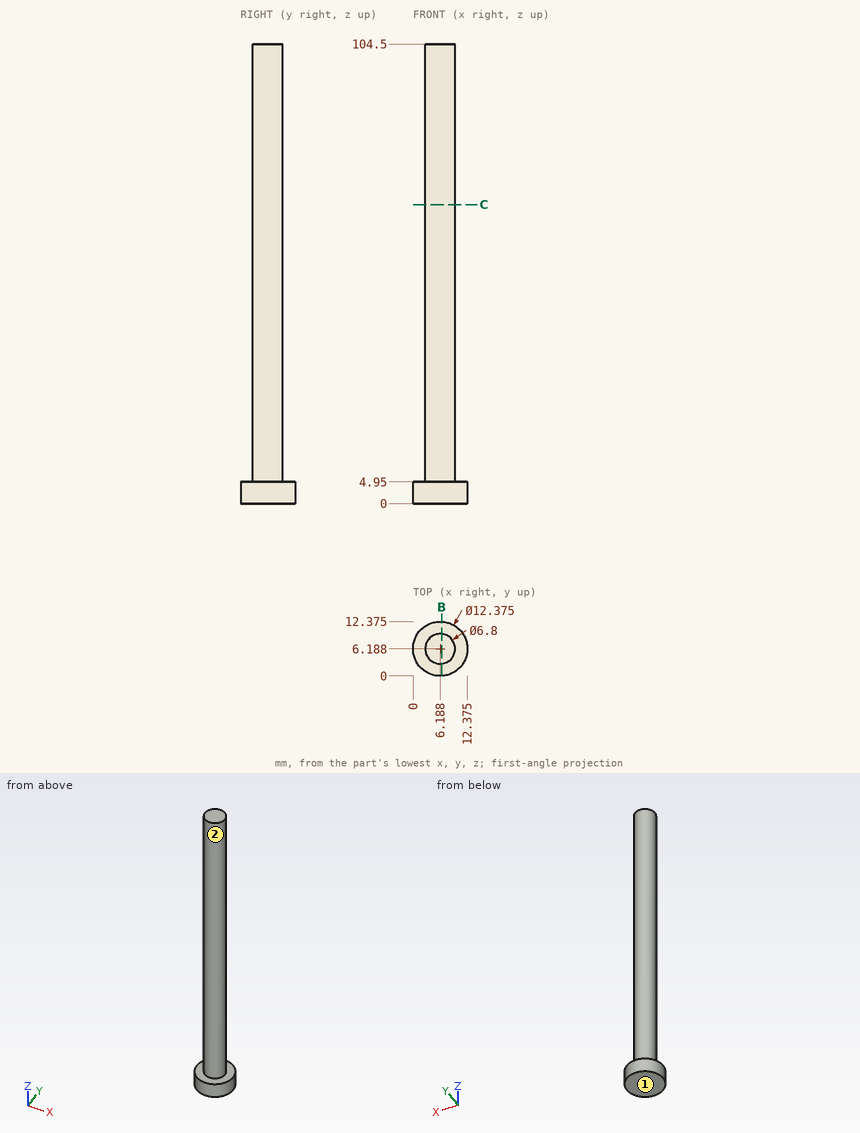
Geometry check sheet. Reference: drawing and pictorial views, mm from the part's lowest x, y, z. A direction names the side the tool comes from. Give positions to 0.01 mm unless a question says otherwise; leave off trailing zeros. Write each loop counter-clockwise with the first axis right and the second up, starting at its lowest first coordinate (ties: lowest second). Pieces come first, ordered by that corner, then holes. Notation, with made-up numbers: (-26, -12.5) -> (-3, -12.5) arc R25 cw to (-3, 0.5) -> close; hole circle Ø1 at (20, -33). An arc over 180 degrees is marked (long way). One line per item, written item: value. Start each with the question number.
Item 1: Section check C-C on z = 68. Record the cut outline in (x, y).
Item 2: Section check B-B on x = 6.5. Record the cut outline in (y, z), then the cut area to 3 significant figures.
Item 3: Material ranges on probe 1 along Z at (x, y) = (0.5, 7.25); probe 2 along X at (y, z) = (6.5, 62); probe 3 along X at (y, z) = (3.5, 66) (1 decimal), recorded low to high. Write a range as from..to.
Item 4: Gauge pin test, flat ends, axial feed: pin 1 (5 mm diameter, centred on x = 3.5, z = 33.5, fed in from +Y); pin 2 (3 mm diameter, centred on y = 6, z = 48, fed in from -X); pin 3 (6 mm diameter, centred on y = 1.5, z = 38.5, fed in from +X). Record the tip position at first contact, or that the pin passes through.
Item 5: Tool access check on the marked faces 1 and 2. Record the directions out of +Z, -Z, +X, -X, +Y, -Y that give a thin tool (end or side, any length) a straight path to the whole face; none if there is none.
Results list:
1. outline: circle Ø6.8 at (6.19, 6.19)
2. outline: (0.01, 0) -> (12.37, 0) -> (12.37, 4.95) -> (9.57, 4.95) -> (9.57, 104.5) -> (2.8, 104.5) -> (2.8, 4.95) -> (0.01, 4.95) -> close
2. area: 735 mm²
3. probe 1: 0..4.95
3. probe 2: 2.8..9.57
3. probe 3: 4.1..8.3
4. pin 1: y = 9.58
4. pin 2: x = 2.79
4. pin 3: x = 9.14
5. face 1: -Z, +X, -X, +Y, -Y
5. face 2: +Z
